Build history of the part. All positions in model axes, mm. A direction names the side the tool comes from. Round coordinates to 2 decimals unless told otherwise and drop trailing zeros. Loops run counter-clockwise (first coordinate to the right, second up) from the corner with the lowest first, then second, coordinate; pieces in that order, holes last. Notation, with made-up numbers: (54.5, -3) - (112.5, -3) arc R33 ccw to (112.5, 34) - close; hole circle Ø4 at (-7.5, 54). An arc over 180 degrees is marked (long way). One line per question, with ' | ' between items. Start each with the question number.
from build123d import *

# Parameters (mm, degrees)
SKETCH_R  = 50
PAD_DEPTH = 2


with BuildPart() as part:
    # Sketch → Pad (new body)
    with BuildSketch(Plane.XY):
        Circle(SKETCH_R)
        with BuildLine():
            ThreePointArc((-1, 47.989582), (-41.569219, 24), (-42.060197, -23.128766))
            Line((-42.060197, -23.128766), (-37.73007, -20.628766))
            Line((-37.73007, -20.628766), (-36.73007, -22.360817))
            Line((-36.73007, -22.360817), (-41.060197, -24.860817))
            ThreePointArc((-41.060197, -24.860817), (0, -48), (41.060197, -24.860817))
            Line((41.060197, -24.860817), (32.399943, -19.860817))
            Line((32.399943, -19.860817), (33.399943, -18.128766))
            Line((33.399943, -18.128766), (42.060197, -23.128766))
            ThreePointArc((42.060197, -23.128766), (41.569219, 24), (1, 47.989582))
            Line((1, 32.989582), (1, 47.989582))
            Line((-1, 32.989582), (1, 32.989582))
            Line((-1, 47.989582), (-1, 32.989582))
        make_face(mode=Mode.SUBTRACT)
    extrude(amount=PAD_DEPTH)


solid = part.part
1) Saw through at B-B on z = 1.5. Write the cut outline in (x, y).
2) Saw through at C-C on x = 24. Write the cut outline in (y, z), and give its area (3 significant figures).
3) Saw through at A-A on y = 39. Write the cut outline in (x, z), and give its area (3 significant figures).
4) Tool access for faces 4 (the cylindrical face through (-41.22, 24.595, 0.986)), 5 (the flat face through (0, 34, 2)): list every direction of +Z, -Z, +X, -X, +Y, -Y with a clear straight run to the whole face (end or side of a thin tool).
5) Wall check: line 1 (Y direction, x = -40.5, z = 1.6); line 2 (Y direction, x = 36, z = 1.2); line 3 (X direction, y = 1, z = 1.2). Give the ranges that are in metal, low to high. Write a range as [from, to].
6) Saw through at D-D on y = 22. Write the cut outline in (x, z), and give its area (3 significant figures).
7) Two-plate mould, pull along X, no slides. Class faces 1 (the flat face through (-39.93, -21.9, 0.99)), 2 (the flat face through (0, 34, 0)), 3 (the cylindrical face through (47.69, 15.02, 0.99)): +X half, -X half, draft (parallel to the pull), parting line (faces both ways), or undercut.
Answer key:
1) outline: circle Ø100 at (0, 0); hole (-42.06, -23.13) - (-37.73, -20.63) - (-36.73, -22.36) - (-41.06, -24.86) arc R48 ccw to (41.06, -24.86) - (32.4, -19.86) - (33.4, -18.13) - (42.06, -23.13) arc R48 ccw to (1, 47.99) - (1, 32.99) - (-1, 32.99) - (-1, 47.99) arc R48 ccw to start
2) outline: (-43.86, 0) - (-41.57, 0) - (-41.57, 2) - (-43.86, 2) - close; (41.57, 0) - (43.86, 0) - (43.86, 2) - (41.57, 2) - close | area: 9.18 mm²
3) outline: (-31.29, 0) - (-27.98, 0) - (-27.98, 2) - (-31.29, 2) - close; (-1, 0) - (1, 0) - (1, 2) - (-1, 2) - close; (27.98, 0) - (31.29, 0) - (31.29, 2) - (27.98, 2) - close | area: 17.2 mm²
4) face 4: +Z, -Z | face 5: +Z, +X, -X, +Y, -Y
5) line 1: [-29.32, -25.76], [-24.54, -22.23], [25.76, 29.32] | line 2: [-34.7, -31.75], [-21.94, -19.63], [31.75, 34.7] | line 3: [-49.99, -47.99], [47.99, 49.99]
6) outline: (-44.9, 0) - (-42.66, 0) - (-42.66, 2) - (-44.9, 2) - close; (42.66, 0) - (44.9, 0) - (44.9, 2) - (42.66, 2) - close | area: 8.95 mm²
7) face 1: undercut | face 2: draft | face 3: parting line
